Check sheet for the modelled part. Datum: model origin and axes. Units: mm. A direction names the side the tool comes from. Coordinates: 2 decimals unless noted, no trailing zeros. Loops run counter-clockwise (first coordinate to the right, second up) from the corner with the lowest first, then second, coordinate; pieces in that order, holes last. Notation, with made-up numbers: (43.5, 11.5) - (74.5, 11.5) arc R18 ccw to (74.5, 25.5) - close; hole circle Ø4 at (-33, 54.25). An arc over 180 degrees is marked (long way). Use a Markdown table: item, result. Add a question column.
1) Draft check along Z on faces 3 (the flat face through (18.3, 2.5, -8.5)), 4 (the cylindrical face through (-25.296, 4.528, -16.128)), 5 (the flat face through (20, -6.5, 6)). Enter one of: pulls with the +Z half, pulls with the -Z half, needs draft (parallel to the pull), parting line crosses it, or undercut.
2) Thickness scan on line 1 (X direction, y = -5.5, z = 0); line 2 (Y direction, x = -16, z = 24); line 3 (Z direction, x = -6.5, y = -2). Record the ranges inside material, lowest first.
3) Sectioned sample at B-B, the plane y = 1. Enter the section's corners in (x, z).
4) Sectioned sample at A-A, the plane y = 5. Enter the section's corners in (x, z).
5) Tool access check on faces 1 (the flat face through (20, 6.5, -6)), 2 (the flat face through (27, -2.5, -9)). Record the directions out of +Z, -Z, +X, -X, +Y, -Y that give a thin tool (end or side, any length) a straight path to the whole face; none if there is none.
6) Go/stop test with flat-tipped pins: P1, Ø3, axis at x = -20.5, y = -3, coming from the -Z side; P2, Ø5, axis at x = -17, z = -5, coming from the -Y side; P3, Ø3, axis at x = -4, z = -18, coming from the -Y side. Record where each tip stops, or that it passes through.
from build123d import *
from build123d.topology import SkipClean


with BuildPart() as part:
    # Sketch1 → Revolve1 (revolve)
    with SkipClean():  # the faces are left unmerged after this step: merging them gives an invalid solid
        with BuildSketch(Plane.XY, mode=Mode.PRIVATE) as revolve1_sk:
            with BuildLine():
                Line((20, 6.5), (20, 2.5))
                Line((20, 2.5), (22.550510257, 2.5))
                ThreePointArc((22.550510257, 2.5), (25, 3.5), (27.449489743, 2.5))
                Line((27.449489743, 2.5), (30, 2.5))
                Line((30, 2.5), (30, 6.5))
                Line((30, 6.5), (20, 6.5))
            make_face()
            with BuildLine():
                Line((27.449489743, 2.5), (22.550510257, 2.5))
                ThreePointArc((22.550510257, 2.5), (21.5, 0), (22.550510257, -2.5))
                Line((22.550510257, -2.5), (27.449489743, -2.5))
                ThreePointArc((27.449489743, -2.5), (28.226702194, -1.355873501), (28.5, 0))
                ThreePointArc((28.5, 0), (28.226702194, 1.355873501), (27.449489743, 2.5))
            make_face()
            with BuildLine():
                ThreePointArc((27.449489743, 2.5), (25, 3.5), (22.550510257, 2.5))
                Line((22.550510257, 2.5), (27.449489743, 2.5))
            make_face()
            with BuildLine():
                Line((27.449489743, -2.5), (22.550510257, -2.5))
                ThreePointArc((22.550510257, -2.5), (25, -3.5), (27.449489743, -2.5))
            make_face()
            with BuildLine():
                Line((22.550510257, -2.5), (20, -2.5))
                Line((20, -2.5), (20, -6.5))
                Line((20, -6.5), (30, -6.5))
                Line((30, -6.5), (30, -2.5))
                Line((30, -2.5), (27.449489743, -2.5))
                ThreePointArc((27.449489743, -2.5), (25, -3.5), (22.550510257, -2.5))
            make_face()
        revolve(revolve1_sk.sketch.rotate(Axis((0, 0, 0), (0, 1, 0)), 90), axis=Axis((0, 0, 0), (0, 1, 0)))


solid = part.part
Solved:
| question | item | result |
|---|---|---|
| 1 | face 3 | undercut |
| 1 | face 4 | parting line crosses it |
| 1 | face 5 | needs draft |
| 2 | line 1 | x = -30 to -20, 20 to 30 |
| 2 | line 2 | y = -6.5 to -2.5, 2.5 to 6.5 |
| 2 | line 3 | z = -27.1 to -21.15, 21.15 to 27.1 |
| 3 | outline | circle Ø56.71 at (0, 0); hole circle Ø43.29 at (0, 0) |
| 4 | outline | circle Ø60 at (0, 0); hole circle Ø40 at (0, 0) |
| 5 | face 1 | +Z, -Z, +X, -X, +Y |
| 5 | face 2 | none |
| 6 | P1 | stops at z = -23.22 |
| 6 | P2 | stops at y = -6.5 |
| 6 | P3 | passes through |
